```python
from build123d import *

# Parameters (mm, degrees)
BOSS_EXTRUDE1_DEPTH = 3


with BuildPart() as part:
    # Sketch1 → Boss-Extrude1 (new body)
    with BuildSketch(Plane.XY):
        with BuildLine():
            Line((-20, -42), (-20, -38))
            Line((-20, -38), (-60, -38))
            Line((-60, -38), (-60, -42))
            Line((-60, -42), (-100, -42))
            Line((-100, -42), (-100, 42))
            Line((-100, 42), (-9.4, 42))
            Line((-9.4, 42), (-9.4, 29.437955396))
            ThreePointArc((-9.4, 29.437955396), (-8.65, 27.879616867), (-7.9, 29.437955396))
            Line((-7.9, 29.437955396), (-7.9, 45.839266813))
            ThreePointArc((-7.9, 45.839266813), (-8.192893219, 46.546373594), (-8.9, 46.839266813))
            Line((-8.9, 46.839266813), (-9, 46.839266813))
            ThreePointArc((-9, 46.839266813), (-9.707106781, 47.132160032), (-10, 47.839266813))
            Line((-10, 47.839266813), (-10, 47.939266813))
            ThreePointArc((-10, 47.939266813), (-9.707106781, 48.646373594), (-9, 48.939266813))
            Line((-9, 48.939266813), (-1, 48.939266813))
            Line((-1, 48.939266813), (-1, 27.583372359))
            ThreePointArc((-1, 27.583372359), (0, 25.749782911), (1, 27.583372359))
            Line((1, 27.583372359), (1, 48.939266813))
            Line((1, 48.939266813), (9, 48.939266813))
            ThreePointArc((9, 48.939266813), (9.707106781, 48.646373594), (10, 47.939266813))
            Line((10, 47.939266813), (10, 47.839266813))
            ThreePointArc((10, 47.839266813), (9.707106781, 47.132160032), (9, 46.839266813))
            Line((9, 46.839266813), (8.9, 46.839266813))
            ThreePointArc((8.9, 46.839266813), (8.192893219, 46.546373594), (7.9, 45.839266813))
            Line((7.9, 45.839266813), (7.9, 29.437955396))
            ThreePointArc((7.9, 29.437955396), (8.65, 27.879616867), (9.4, 29.437955396))
            Line((9.4, 29.437955396), (9.4, 42))
            Line((9.4, 42), (100, 42))
            Line((100, 42), (100, -42))
            Line((100, -42), (60, -42))
            Line((60, -42), (60, -38))
            Line((60, -38), (20, -38))
            Line((20, -38), (20, -42))
            Line((20, -42), (-20, -42))
        make_face()
    extrude(amount=BOSS_EXTRUDE1_DEPTH)


solid = part.part
```
For this review, take the finished solid that the model builds, in its own axes (mm). Give positions to 0.01 mm unless a question says otherwise; leave off trailing zeros. Loops run counter-clockwise (first coordinate to the right, second up) from the corner with the lowest first, then second, coordinate; pieces in that order, holes last. Notation, with made-up numbers: M 54.5,-12.5 L 77.5,-12.5 A7 ccw 77.5,-8.5 Z; hole C 20.25,24 d5. An arc over 180 degrees is marked long. One line per item, written item: value. Start each with the question number.
Q1. Add section B-B (x = -50). Give the boundary of the cut face in (y, z), and give its area (3 significant figures).
Q2. Clearance check with flat-ended pins moving along their axes: pin 1 Ø1.5 at (x, z) = (44.5, 2) entering from -Y; pin 2 Ø1.5 at (x, y) = (8.65, 28.84) entering from +Z; pin 3 Ø1.5 at (x, z) = (-58, 1.5) entering from +Y. State where each tip first meets the part, or that it passes through.
Q3. Add section C-C (x = -75). Give the boundary of the cut face in (y, z).
Q4. For L1, parallel to X at y = 38.5, z = 1.75; L2, parallel to Y at x = 8.65, z = 0.95; L3, parallel to Y at x = -75, z = 0.2, list the stretches that pass through material, from the lowest coordinate up.
Reply:
1. outline: M -38,0 L 42,0 L 42,3 L -38,3 Z
1. area: 240 mm²
2. pin 1: y = -38
2. pin 2: through
2. pin 3: y = 42
3. outline: M -42,0 L 42,0 L 42,3 L -42,3 Z
4. L1: -100 to -9.4, -7.9 to -1, 1 to 7.9, 9.4 to 100
4. L2: -42 to 27.88, 46.81 to 48.94
4. L3: -42 to 42
